Verification items for the finished model (mm, model axes). Face numbers are marked on the shaded views. A direction names the side the tool comes from. Round coordinates to 2 decimals unless told otherwise and drop trailing zeros. Order: outer loops, then holes, each group sorted by start corner. A loop starts at its lowest first (then second) coordinate and runs counter-clockwise, first axis right, second up. Notation, with made-up numbers: (85.25, -13) -> (117.25, -13) arc R11 cw to (117.25, -9) -> close; hole circle Ø10 at (31, 79). An arc over 180 degrees is marked (long way). Put each result on its own line as item: value.
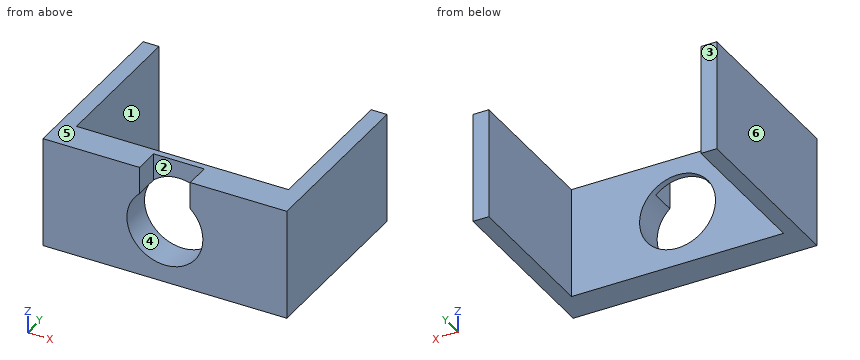
```python
from build123d import *

# Parameters (mm, degrees)
EXTRUSION1_DEPTH = 35
ESQUISSE2_R      = 12
EXTRUSION2_DEPTH = 58
EXTRUSION3_DEPTH = 8


with BuildPart() as part:
    # Esquisse1 → Extrusion1 (new body)
    with BuildSketch(Plane.XY):
        Polygon((72, -57), (72, 0), (67, 0), (67, -47), (0, -47), (0, 0), (-5, 0), (-5, -57), align=None)
    extrude(amount=EXTRUSION1_DEPTH)

    # Esquisse2 → Extrusion2 (cut, through all)
    with BuildSketch(Plane.XZ.offset(57)):
        with Locations((33.5, 17.5)):
            Circle(ESQUISSE2_R)
    extrude(amount=-EXTRUSION2_DEPTH, mode=Mode.SUBTRACT)

    # Esquisse3 → Extrusion3 (cut)
    with BuildSketch(Plane.XZ.offset(57)):
        with BuildLine():
            Line((41.5, 26.44427191), (41.5, 35))
            Line((41.5, 35), (25.5, 35))
            Line((25.5, 35), (25.5, 26.44427191))
            ThreePointArc((25.5, 26.44427191), (33.5, 29.5), (41.5, 26.44427191))
        make_face()
    extrude(amount=-EXTRUSION3_DEPTH, mode=Mode.SUBTRACT)


solid = part.part
```
Item 1: Sectioned sample at C-C, the plane x = 33.5. Record the boundary of the cut face in (y, z).
Geometry check:
outline: (-57, 0) -> (-47, 0) -> (-47, 5.5) -> (-57, 5.5) -> close; (-49, 29.5) -> (-47, 29.5) -> (-47, 35) -> (-49, 35) -> close
Item 2: Release check for a two-part mould opening along X. For the marked faces 4, 5 and 6 record: pulls with the +X half, pulls with the -X half, needs draft (parallel to the pull), parting line crosses it, or undercut.
Geometry check:
face 4: undercut
face 5: needs draft
face 6: pulls with the -X half
Item 3: Tool access check on the marked faces 1, 2 and 3. Record the directions out of +Z, -Z, +X, -X, +Y, -Y that give a thin tool (end or side, any length) a straight path to the whole face; none if there is none.
Geometry check:
face 1: +Z, -Z, +Y
face 2: +Z, -Y
face 3: +Z, -Z, +X, -X, +Y
Item 4: Depth check by flat-ended pin: pin 1 Ø9.5 at (x, z) = (30.5, 29.5) entering from -Y; pin 2 Ø3 at (x, z) = (10, 27.5) entering from +Y. Enter the tip coordinate at first touch or a pass-through.
Geometry check:
pin 1: y = -49
pin 2: y = -47
Item 5: Sectioned sample at D-D, the plane y = -50.5. Record the boundary of the cut face in (x, z).
Geometry check:
outline: (-5, 0) -> (72, 0) -> (72, 35) -> (41.5, 35) -> (41.5, 26.44) arc R12 cw (long way) to (25.5, 26.44) -> (25.5, 35) -> (-5, 35) -> close
Item 6: Material ranges on line 1 along X through (y, z) = (-53, 17); line 2 along X through (y, z) = (-21, 31); line 3 along Y through (x, z) = (14.5, 23), recorded low to high.
Geometry check:
line 1: -5 to 21.51, 45.49 to 72
line 2: -5 to 0, 67 to 72
line 3: -57 to -47
Item 7: Sectioned sample at B-B, the plane y = -41.5. Record the boundary of the cut face in (x, z), then the cut area to 3 significant figures.
Geometry check:
outline: (-5, 0) -> (0, 0) -> (0, 35) -> (-5, 35) -> close; (67, 0) -> (72, 0) -> (72, 35) -> (67, 35) -> close
area: 350 mm2
Item 8: Sectioned sample at A-A, the plane z = 17.5. Record the boundary of the cut face in (x, y).
Geometry check:
outline: (-5, -57) -> (21.5, -57) -> (21.5, -47) -> (0, -47) -> (0, 0) -> (-5, 0) -> close; (45.5, -57) -> (72, -57) -> (72, 0) -> (67, 0) -> (67, -47) -> (45.5, -47) -> close
